Design review of the part built by this model. Coordinates are the model's own, in mm. Face numbers are marked on the shaded views. A direction names the side the tool comes from. Give positions to 0.01 mm unless a question says otherwise; leave off trailing zeros. Loops run counter-clockwise (first coordinate to the right, second up) from the corner with the lowest first, then second, coordinate; pieces in that order, holes last.
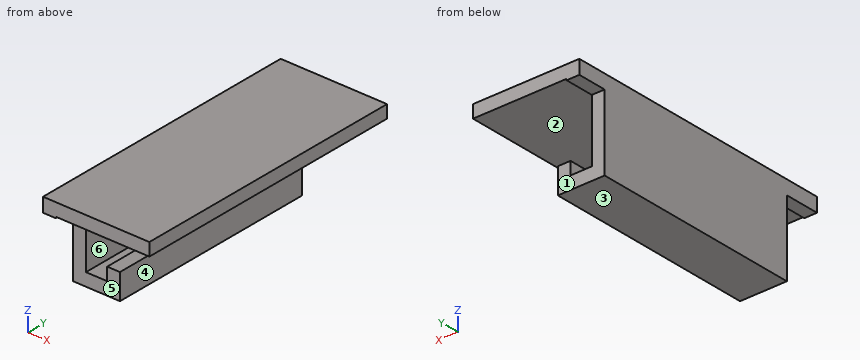
from build123d import *

# Parameters (mm, degrees)
F1_DEPTH = 65.2
F3_DEPTH = 25


with BuildPart() as f1:
    # F0 (on Front) → F1 (new body)
    with BuildSketch(Plane.XZ):
        Polygon((-27.608158, 12), (-27.608158, 15), (-62.608158, 15), (-62.608158, -6), (-51.608158, -6), (-51.608158, 0), (-54.608158, 0), (-54.608158, -3), (-59.608158, -3), (-59.608158, 12), align=None)
    extrude(amount=F1_DEPTH)

    # F2 (on face) → F3 (intersect)
    with BuildSketch(Plane(origin=(-62.608158, 0, 0), x_dir=(0, -1, 0), z_dir=(-1, 0, 0))):
        Polygon((0, 15), (0, 11.699338), (6.923881, 11.699338), (6.923881, -6), (32.6, -6), (56.923881, -6), (56.923881, 11.699338), (65.2, 11.699338), (65.2, 15), align=None)
    extrude(amount=-F3_DEPTH, mode=Mode.INTERSECT)


solid = f1.part
Q1. Take a section at B-B (y = -5.5). Give the boundary of the cut face in (x, z).
Results:
outline: (-62.61, 11.7) - (-59.61, 11.7) - (-59.61, 12) - (-37.61, 12) - (-37.61, 15) - (-62.61, 15) - close
Q2. Take a section at D-D (z = 2). Give the boundary of the cut face in (x, y), plus the area to 3 significant figures.
Results:
outline: (-62.61, -56.92) - (-59.61, -56.92) - (-59.61, -6.92) - (-62.61, -6.92) - close
area: 150 mm2
Q3. Insertion check: pin 1 (12 mm diameter, centred on x = -54.5, z = 6.5, fed in from -Y); pin 2 (9 mm diameter, centred on x = -58.5, z = 0, fed in from -Y); pin 3 (3 mm diameter, centred on y = -22.5, z = -4, fed in from +X); pin 4 (2 mm diameter, centred on x = -44, y = -37.5, fed in from -Z). Each pin has a flat end and moves straight along its axis. Give the tip position at first contact, or say it passes through.
Results:
pin 1: stops at y = -65.2
pin 2: stops at y = -56.92
pin 3: stops at x = -51.61
pin 4: stops at z = 12
Q4. Take a section at A-A (x = -52.25). Give the boundary of the cut face in (y, z), plus the area to 3 significant figures.
Results:
outline: (-65.2, 12) - (0, 12) - (0, 15) - (-65.2, 15) - close; (-56.92, -6) - (-6.92, -6) - (-6.92, 0) - (-56.92, 0) - close
area: 496 mm2
Q5. Wall thickness on line 1 (Z direction, x = -55.5, y = -7.5); line 2 (Z direction, x = -53.25, y = -47); line 3 (Z direction, x = -50.5, y = -56): over which ranges is each line inside the solid? List them lowest first.
Results:
line 1: z = -6 to -3, 12 to 15
line 2: z = -6 to 0, 12 to 15
line 3: z = 12 to 15
Q6. Draft analysis for pull direction X (two halves, no side actions). For the marked faces 4, 5 and 6, state which applies: pulls with the +X half, pulls with the -X half, needs draft (parallel to the pull), parting line crosses it, or undercut.
Results:
face 4: pulls with the +X half
face 5: needs draft
face 6: undercut
Q7. Tool access review of the marked faces 1, 2 and 3: name each direction out of +Z, -Z, +X, -X, +Y, -Y from which nothing blocks a thin tool from reaching the whole face with its end or side.
Results:
face 1: -Z, +X, -X, +Y
face 2: +X, +Y, -Y
face 3: -Z, +X, -X, +Y, -Y
Q8. Take a section at C-C (x = -57.5). Give the boundary of the cut face in (y, z), plus the area to 3 significant figures.
Results:
outline: (-65.2, 12) - (0, 12) - (0, 15) - (-65.2, 15) - close; (-56.92, -6) - (-6.92, -6) - (-6.92, -3) - (-56.92, -3) - close
area: 346 mm2
